from build123d import *

# Parameters (mm, degrees)
F1_DEPTH = 52.88097
F2_R     = 5.629774
F3_DEPTH = 25.4
F4_W     = 21.416974
F4_H     = 30.958728
F5_DEPTH = 10.13054
F7_DEPTH = 25


with BuildPart() as f1:
    # F0 (on Top) → F1 (new body)
    with BuildSketch(Plane.XY):
        Polygon((-32.995568, -19.05), (0, 0), (-32.995568, 19.05), align=None)
    extrude(amount=F1_DEPTH)

    # F2 (on face) → F3 (cut)
    with BuildSketch(Plane.XY.offset(52.88097)):
        with Locations((-21.997045, 0)):
            Circle(F2_R)
    extrude(amount=-F3_DEPTH, mode=Mode.SUBTRACT)

    # F4 (on face) → F5 (cut)
    with BuildSketch(Plane(origin=(-32.995568, 0, 0), x_dir=(0, -1, 0), z_dir=(-1, 0, 0))):
        with Locations((0, 26.440485)):
            Rectangle(F4_W, F4_H)
    extrude(amount=-F5_DEPTH, mode=Mode.SUBTRACT)

    # F6 (on face) → F7 (cut)
    with BuildSketch(Plane.XY.offset(52.88097)):
        Polygon((-24.02568, -9.358168), (-28.524186, -6.694105), (-26.91254, -10.997219), align=None)
    extrude(amount=-F7_DEPTH, mode=Mode.SUBTRACT)


solid = f1.part
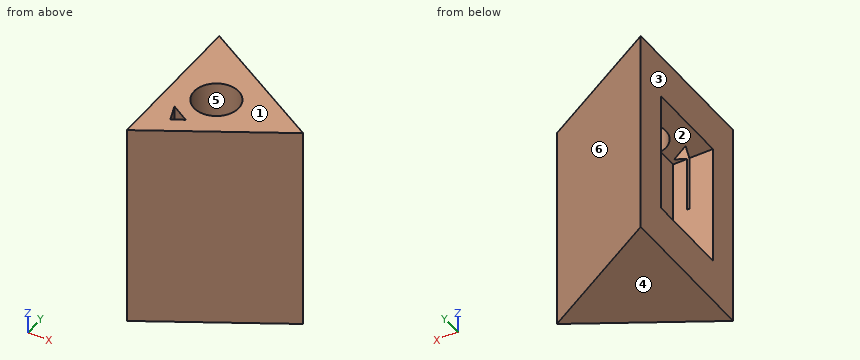
The listing builds one solid part. Answer for the finished solid, in the listing's coordinates (mm). Face numbers are marked on the shaded views. A direction names the side the tool comes from. Give positions to 0.01 mm unless a question says otherwise; leave off trailing zeros. Write each loop counter-clockwise with the first axis right and the second up, starting at its lowest first coordinate (ties: lowest second). Pieces come first, ordered by that corner, then holes.
Item 1: Which of the six approach directions +Z, -Z, +X, -X, +Y, -Y give full straight-line access (tool end or side, diameter ignored) to the marked faces 1 and 2?
Item 2: Flat-ended cylindrical pins translate along their axes: P1, Ø1.5, axis at x = -8, z = 13.5, coming from the +Y side; P2, Ø10, axis at x = -23.5, z = 10.5, coming from the -Y side; P3, Ø1.9, axis at x = -20.5, y = -3, coming from the +Z side. Find the tip coordinate at first contact, or state that the pin passes through.
Item 3: Section C-C, the plane x = -30 is taken. Write down the section's boundary in (y, z).
Item 4: Section D-D, the plane y = -3.5 is taken. Write down the section's boundary in (x, z), plus the area to 3 significant figures.
Item 5: Section A-A, the plane z = 43.5 is taken. Write down the section's boundary in (x, y), plus the area to 3 significant figures.
Item 6: Find the intervals of material crossed by line 1 along Z through (x, y) = (-31, 2); line 2 along Y through (x, z) = (-17, 36); line 3 along X through (y, z) = (-7.5, 42), in increasing order.
Item 7: Determine the mould class of the marked faces 3, 4, 5 and 6 for opening direction X: released by +X, released by -X, zero draft, split by the parting line, or undercut.
Item 8: Section B-B, the plane y = 2.5 is taken. Write down the section's boundary in (x, z).
Completed:
1. face 1: +Z, +X, -X, +Y, -Y
1. face 2: -X
2. P1: stops at y = 5.05
2. P2: stops at y = -16.45
2. P3: stops at z = 27.48
3. outline: (-17.32, 0) - (17.32, 0) - (17.32, 52.88) - (-17.32, 52.88) - close; hole (-10.71, 10.96) - (10.71, 10.96) - (10.71, 41.92) - (-10.71, 41.92) - close
4. outline: (-33, 0) - (-6.06, 0) - (-6.06, 52.88) - (-17.59, 52.88) - (-17.59, 27.48) - (-22.87, 27.48) - (-22.87, 10.96) - (-33, 10.96) - close; (-33, 41.92) - (-26.41, 41.92) - (-26.41, 52.88) - (-33, 52.88) - close
4. area: 938 mm2
5. outline: (-33, -19.05) - (0, 0) - (-33, 19.05) - close; hole (-28.52, -6.69) - (-26.91, -11) - (-24.03, -9.36) - close; hole circle Ø11.26 at (-22, 0)
5. area: 521 mm2
6. line 1: z = 0 to 10.96, 41.92 to 52.88
6. line 2: y = -9.81 to -2.59, 2.59 to 9.81
6. line 3: x = -33 to -28.22, -27.16 to -12.99
7. face 3: released by -X
7. face 4: zero draft
7. face 5: undercut
7. face 6: released by +X
8. outline: (-33, 0) - (-4.33, 0) - (-4.33, 52.88) - (-16.95, 52.88) - (-16.95, 27.48) - (-22.87, 27.48) - (-22.87, 10.96) - (-33, 10.96) - close; (-33, 41.92) - (-27.04, 41.92) - (-27.04, 52.88) - (-33, 52.88) - close
